Source: CAD feature listing. Evaluate the final solid. Frame: model axes, mm. Face numbers are marked on the shaded views. A direction names the side the tool comes from. Round coordinates to 2 decimals unless told otherwise and drop trailing zeros. Loops run counter-clockwise (first coordinate to the right, second up) from the corner with the lowest first, then second, coordinate; pieces in that order, holes last.
(1) Section B-B, the plane y = 5.5. Return the cut outline in (x, z).
(2) Material intervals for probe 1 along Y at (x, z) = (1, 1); probe 2 along Y at (x, z) = (0, -2.5); probe 3 along Z at (x, y) = (-0.25, 0.75), sorted ascending.
(3) Mould query, pull axis Z, two halves, no side actions, for the marked faces 4, 5 and 6. Classes: pulls with the +Z half, pulls with the -Z half, needs draft (parallel to the pull), parting line crosses it, or undercut.
(4) Set-up query: the marked faces 1, 2 and 3. Return all of +Z, -Z, +X, -X, +Y, -Y with unobstructed straight access to the full face (end or side cutting, diameter ignored); none if empty.
(5) First-contact query: pin 1 Ø1 at (x, z) = (2.5, -1) entering from +Y; pin 2 Ø2 at (x, z) = (2, 3) entering from +Y; pin 3 Ø0.8 at (y, z) = (0.5, 0) entering from -X. Flat tips, straight axial feed; report the tip coordinate or a pass-through.
```python
from build123d import *

# Parameters (mm, degrees)
SKETCH1_R           = 4
BOSS_EXTRUDE1_DEPTH = 2
SKETCH2_R           = 1.95
BOSS_EXTRUDE2_DEPTH = 6
CHAMFER1_SIZE       = 2
CUT_EXTRUDE1_DEPTH  = 1.5


with BuildPart() as part:
    # Sketch1 → Boss-Extrude1 (new body)
    with BuildSketch(Plane(origin=(0, 0, 0), x_dir=(1, 0, 0), z_dir=(0, 1, 0))):
        with Locations(Location((0, 0, 0), (0, 0, 270))):
            Circle(SKETCH1_R)
    extrude(amount=BOSS_EXTRUDE1_DEPTH)

    # Sketch2 → Boss-Extrude2 (add)
    with BuildSketch(Plane(origin=(0, 2, 0), x_dir=(1, 0, 0), z_dir=(0, 1, 0))):
        with Locations(Location((0, 0, 0), (0, 0, 270))):
            Circle(SKETCH2_R)
    extrude(amount=BOSS_EXTRUDE2_DEPTH)

    # Chamfer1
    chamfer1_edges = [part.edges().sort_by_distance(p)[0] for p in [
        (0, 2, -4),
    ]]
    chamfer(chamfer1_edges, length=CHAMFER1_SIZE - 0.0001)  # a hair under: the kernel refuses the full size

    # Sketch3 → Cut-Extrude1 (cut)
    with BuildSketch(Plane.XZ):
        Polygon((0, -1.662470902), (1.439742034, -0.831235451), (1.439742034, 0.831235451), (0, 1.662470902), (-1.439742034, 0.831235451), (-1.439742034, -0.831235451), align=None)
    extrude(amount=-CUT_EXTRUDE1_DEPTH, mode=Mode.SUBTRACT)


solid = part.part
```
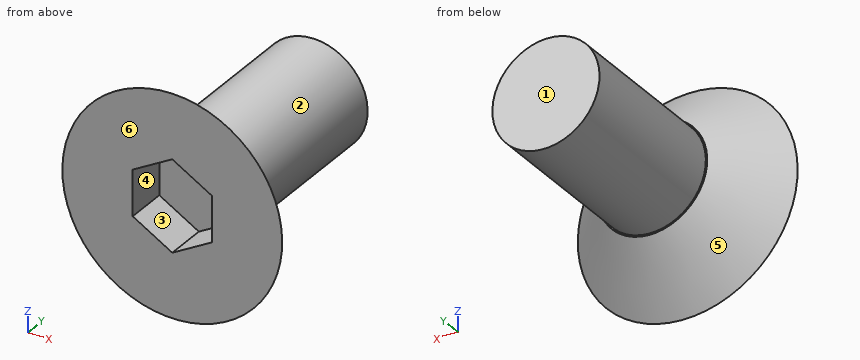
Output values:
1. outline: circle Ø3.9 at (0, 0)
2. probe 1: y = 1.5 to 8
2. probe 2: y = 0 to 1.5
2. probe 3: z = -3.24 to -1.52, 1.52 to 3.24
3. face 4: undercut
3. face 5: parting line crosses it
3. face 6: needs draft
4. face 1: +Z, -Z, +X, -X, +Y
4. face 2: +Y
4. face 3: -Y
5. pin 1: stops at y = 1.81
5. pin 2: stops at y = 1.39
5. pin 3: stops at x = -3.9
